Source: CAD feature listing. Evaluate the final solid. Frame: model axes, mm. Face numbers are marked on the shaded views. A direction names the side the tool comes from. Give positions to 0.01 mm unless a question says otherwise; leave off trailing zeros. Loops run counter-clockwise (first coordinate to the right, second up) from the corner with the lowest first, then second, coordinate; pieces in that order, holes last. Notation, with made-up numbers: M 71,62 L 113,62 A21 cw 113,83 Z; hole C -10.75,74 d2. An arc over 180 degrees is marked long. Answer in a Markdown table with one row per item.
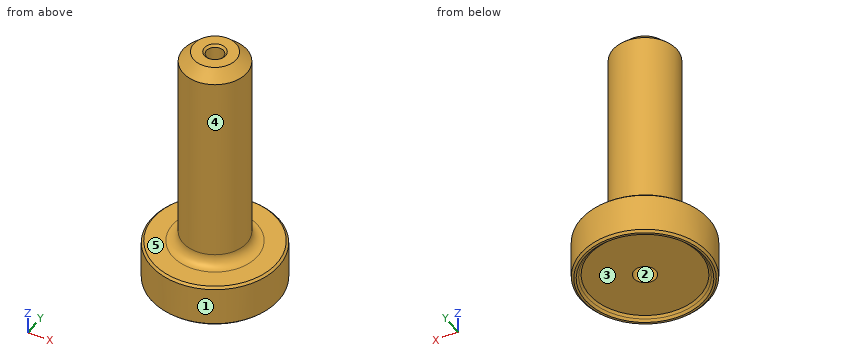
```python
from build123d import *

# Parameters (mm, degrees)
F2_SIZE        = 5
F3_SIZE        = 0.99999
F5_R           = 5
F6_D           = 10.3
F6_DEPTH       = 35.25
F6_TIP         = 3.094432188
F8_D           = 8
F8_DEPTH       = 15
F8_CSINK_D     = 10
F8_CSINK_ANGLE = 90
F8_TIP         = 2.4034424761


# Not quite as in the source:
# - a fillet or chamfer is up to 0.001 mm smaller than in the source, because OpenCascade refuses the exact size


with BuildPart() as f1:
    # F0 (on Front) → F1 (revolve)
    with BuildSketch(Plane.XZ):
        Polygon((-27, 0), (0, 0), (0, 118), (-15, 118), (-15, 18), (-30, 18), (-30, -2), (-27, -2), align=None)
    revolve(axis=Axis((0, 0, 59), (0, 0, -1)))

    # F2
    f2_edges = [f1.edges().sort_by_distance(p)[0] for p in [
        (15, 0, 118),
    ]]
    chamfer(f2_edges, length=F2_SIZE)

    # F3 (size 1 in the source; OpenCascade refuses exactly that, so slightly less here)
    f3_edges = [f1.edges().sort_by_distance(p)[0] for p in [
        (30, 0, 18),
        (30, 0, -2),
        (27, 0, -2),
        (27, 0, 0),
        (-27, 0, -1),
    ]]
    chamfer(f3_edges, length=F3_SIZE)

    # F5
    f5_edges = [f1.edges().sort_by_distance(p)[0] for p in [
        (15, 0, 18),
    ]]
    fillet(f5_edges, radius=F5_R)

    # F6
    with Locations(Plane(origin=(0, 0, 0), x_dir=(1, 0, 0), z_dir=(0, 0, -1))):
        with Locations((0, 0)):
            Hole(F6_D / 2, depth=F6_DEPTH)
            with Locations((0, 0, -(F6_DEPTH + F6_TIP / 2))):  # 118° drill point
                Cone(0, F6_D / 2, F6_TIP, mode=Mode.SUBTRACT)

    # F8
    with Locations(Plane.XY.offset(118)):
        with Locations((0, 0)):
            CounterSinkHole(F8_D / 2, F8_CSINK_D / 2, depth=F8_DEPTH, counter_sink_angle=F8_CSINK_ANGLE)
            with Locations((0, 0, -(F8_DEPTH + F8_TIP / 2))):  # 118° drill point
                Cone(0, F8_D / 2, F8_TIP, mode=Mode.SUBTRACT)


solid = f1.part
```
1) Pull-direction query (Y, two-part tool) for the marked faces 3, 4 and 5; classes: released by +Y, released by -Y, zero draft, split by the parting line, or undercut.
Reply:
| item | result |
|---|---|
| face 3 | undercut |
| face 4 | split by the parting line |
| face 5 | zero draft |
2) Material intervals for L1, parallel to Y at x = 0, z = 24; L2, parallel to Y at x = 0, z = 12.5; L3, parallel to Z at x = -11, y = 26.5, sorted ascending.
Reply:
| item | result |
|---|---|
| L1 | y = -15 to -5.15, 5.15 to 15 |
| L2 | y = -30 to -5.15, 5.15 to 30 |
| L3 | z = -2 to 18 |
3) Section B-B, the plane z = 69. Return loops of the section in (x, y), then the cut area to 3 significant figures.
Reply:
| item | result |
|---|---|
| outline | C 0,0 d30 |
| area | 707 mm² |
4) Pin query (flat end, axial travel): pin 1 Ø5 at (x, y) = (17, -11) entering from -Z; pin 2 Ø5 at (x, y) = (-7, -18) entering from +Z; pin 3 Ø5 at (x, y) = (0, 0) entering from +Z. Return the tip coordinate at first contact, or that it passes through.
Reply:
| item | result |
|---|---|
| pin 1 | stops at z = 0 |
| pin 2 | stops at z = 19.15 |
| pin 3 | stops at z = 102.1 |
5) Section A-A, the plane z = 104.5. Return loops of the section in (x, y), then the cut area to 3 significant figures.
Reply:
| item | result |
|---|---|
| outline | C 0,0 d30; hole C 0,0 d8 |
| area | 657 mm² |
6) Set-up query: the marked faces 1 and 2. Return all of +Z, -Z, +X, -X, +Y, -Y with unobstructed straight access to the full face (end or side cutting, diameter ignored); none if empty.
Reply:
| item | result |
|---|---|
| face 1 | +Z, -Z |
| face 2 | -Z |
